Can you work these out from the drawing? Everything is in mm from the part's minimum corner. A direction names the side the tool comes from. Round coordinates to 2 decimals unless told otherwise and drop trailing zeros. Loops run counter-clockwise (first coordinate to the right, second up) from the corner with the lowest first, then second, coordinate; pieces in that order, holes last. Notation, with made-up numbers: M 50.5,31 L 107.5,31 A14 cw 107.5,55 Z; hole C 69.25,87 d8. An arc over 180 degrees is marked long. Return JSON: item names as keys, results as strings. Group by question number.
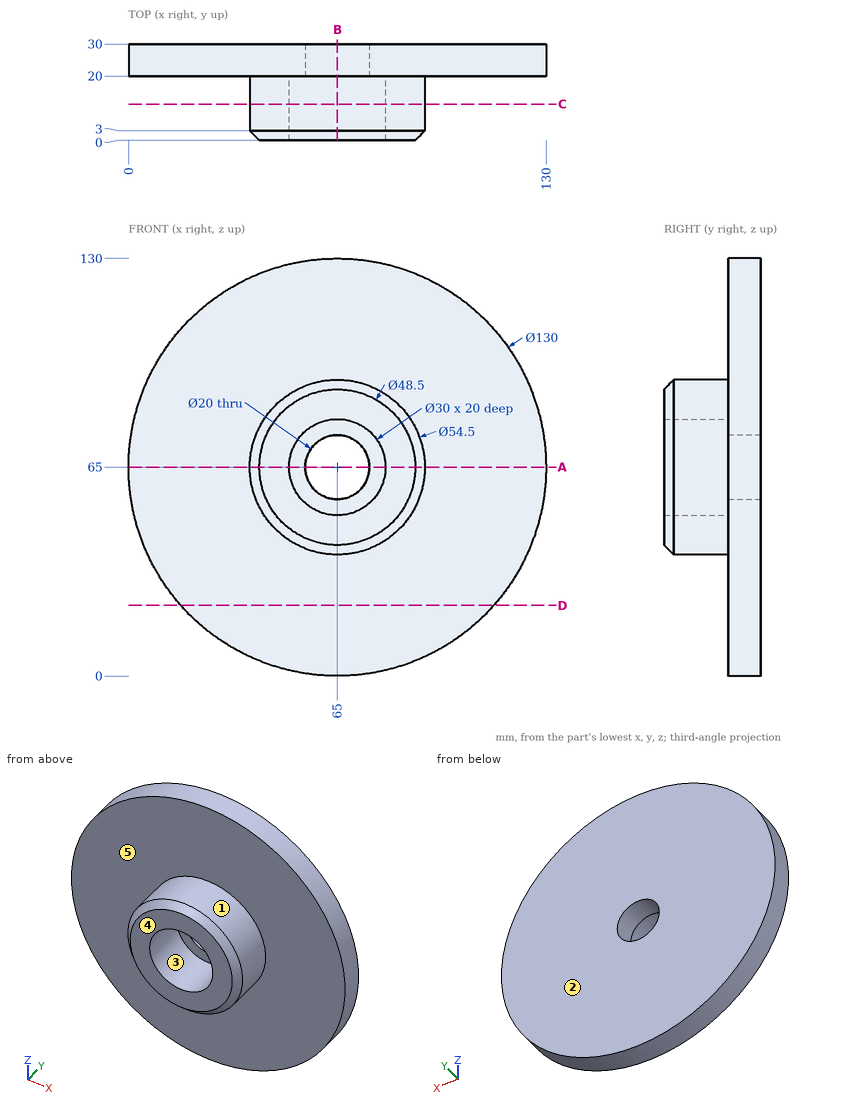
1. If we section it at D-D, the plane z = 22: Please give me the cut outline in (x, y).
2. We'd pull the mould along X, two halves only. Please class the marked faces 1, 2 and 3: +X half, -X half, draft (parallel to the pull), parting line (faces both ways), or undercut.
3. I need wall thicknesses on probe 1 along X at (y, z) = (23, 65); probe 2 along X at (y, z) = (12, 65); probe 3 along Y at (x, z) = (90.5, 37.5). Which ranges of each line are inside material? Lowest first, please.
4. If we section it at A-A, the plane z = 65: Please give me the cut outline in (x, y).
5. If we section it at C-C, the plane y = 11.25: Please give me the cut outline in (x, z), then the cut area to 3 significant figures.
6. I'm going to push flat-ended pins straight in: pin 1 Ø8 at (x, y) = (100, 22.5) entering from +Z; pin 2 Ø10 at (y, z) = (14.5, 44) entering from -X; pin 3 Ø12 at (x, z) = (19.5, 87) entering from -Y. Where does each tip first touch, or does it pass through?
7. If we section it at B-B, the plane x = 65: Please give me the cut outline in (y, z).
8. On a 3-axis mill with a long thin cutter (end or side, diameter ignored), from which of +Z, -Z, +X, -X, +Y, -Y can I reach the whole of each face in a straight line? I mean the marked faces 4 and 5. Say none if no direction works.
Geometry results:
{
 "1": {"outline": "M 16.26,20 L 113.74,20 L 113.74,30 L 16.26,30 Z"},
 "2": {"face 1": "parting line", "face 2": "draft", "face 3": "undercut"},
 "3": {"probe 1": "0 to 55, 75 to 130", "probe 2": "37.75 to 50, 80 to 92.25", "probe 3": "20 to 30"},
 "4": {"outline": "M 0,20 L 37.75,20 L 37.75,3 L 40.75,0 L 50,0 L 50,20 L 55,20 L 55,30 L 0,30 Z; M 75,20 L 80,20 L 80,0 L 89.25,0 L 92.25,3 L 92.25,20 L 130,20 L 130,30 L 75,30 Z"},
 "5": {"outline": "C 65,65 d54.5; hole C 65,65 d30", "area": "1,630 mm^2"},
 "6": {"pin 1": "z = 122.13", "pin 2": "x = 42.94", "pin 3": "y = 20"},
 "7": {"outline": "M 0,40.75 L 3,37.75 L 20,37.75 L 20,0 L 30,0 L 30,55 L 20,55 L 20,50 L 0,50 Z; M 0,80 L 20,80 L 20,75 L 30,75 L 30,130 L 20,130 L 20,92.25 L 3,92.25 L 0,89.25 Z"},
 "8": {"face 4": "+Z, -Z, +X, -X, -Y", "face 5": "-Y"}
}
